```python
from build123d import *

# Parameters (mm, degrees)
SKETCH_1_R               = 13
EXTRUDE_1_DEPTH          = 8
SKETCH_2_R               = 17
EXTRUDE_2_DEPTH          = 8
EXTRUDE_3_DEPTH          = 8
SKETCH_4_R               = 13
EXTRUDE_4_DEPTH          = 6
SKETCH_5_R               = 10
CUT_EXTRUDE_1_DEPTH      = 25
SKETCH_7_R               = 2.5
CUT_EXTRUDE_3_DEPTH      = 32.5
PATTERN_CIRCULAR_1_COUNT = 2


with BuildPart() as part:
    # 草图1 → 凸台-拉伸1 (new body)
    with BuildSketch(Plane.XY):
        Circle(SKETCH_1_R)
    extrude(amount=EXTRUDE_1_DEPTH)

    # 草图2 → 凸台-拉伸2 (add)
    with BuildSketch(Plane(origin=(0, 0, 0), x_dir=(-1, 0, 0), z_dir=(0, 0, -1))):
        Circle(SKETCH_2_R)
    extrude(amount=EXTRUDE_2_DEPTH)

    # 草图3 → 凸台-拉伸3 (add)
    with BuildSketch(Plane.XY.offset(8)):
        with BuildLine():
            Line((2, 17.385338651), (17.385338651, 2))
            ThreePointArc((17.385338651, 2), (17.5, 0), (17.385338651, -2))
            Line((17.385338651, -2), (2, -17.385338651))
            ThreePointArc((2, -17.385338651), (0, -17.5), (-2, -17.385338651))
            Line((-2, -17.385338651), (-17.385338651, -2))
            ThreePointArc((-17.385338651, -2), (-17.5, 0), (-17.385338651, 2))
            Line((-17.385338651, 2), (-2, 17.385338651))
            ThreePointArc((-2, 17.385338651), (0, 17.5), (2, 17.385338651))
        make_face()
    extrude(amount=EXTRUDE_3_DEPTH)

    # 草图4 → 凸台-拉伸4 (add)
    with BuildSketch(Plane.XY.offset(16)):
        Circle(SKETCH_4_R)
    extrude(amount=EXTRUDE_4_DEPTH)

    # 草图5 → 切除-拉伸1 (cut)
    with BuildSketch(Plane(origin=(0, 0, -8), x_dir=(-1, 0, 0), z_dir=(0, 0, -1))):
        Circle(SKETCH_5_R)
    extrude(amount=-CUT_EXTRUDE_1_DEPTH, mode=Mode.SUBTRACT)

    # 草图7 → 切除-拉伸3 (cut)
    with BuildSketch(Plane.XY.offset(22)):
        with Locations((-6, 0)):
            Circle(SKETCH_7_R)
    cut_extrude_3 = extrude(amount=-CUT_EXTRUDE_3_DEPTH, mode=Mode.SUBTRACT)

    # 阵列(圆周)1: 切除-拉伸3 ×2 about axis
    pattern_circular_1_axis = Axis((0, 0, 0), (0, 0, 1))
    for i in range(1, PATTERN_CIRCULAR_1_COUNT):
        add(cut_extrude_3.rotate(pattern_circular_1_axis, i * 360 / PATTERN_CIRCULAR_1_COUNT), mode=Mode.SUBTRACT)


solid = part.part
```
Could you check a few things on this model? Use its own coordinates, in mm. A direction names the side the tool comes from. Coordinates: 2 decimals unless noted, no trailing zeros. Write each loop counter-clockwise with the first axis right and the second up, starting at its lowest first coordinate (ties: lowest second). Pieces come first, ordered by that corner, then holes. Notation, with made-up numbers: (24, 36) - (51, 36) arc R14 cw to (51, 40) - close; hole circle Ø6 at (-26, 7). An arc over 180 degrees is marked (long way). Use a Markdown table: item, result.
Q1. Imagine slicing it at B-B (y = -14). List the corners of the cut face in (x, z) for me, and give its area (3 significant figures).
Geometry check:
| item | result |
|---|---|
| outline | (-9.64, -8) - (9.64, -8) - (9.64, 0) - (-9.64, 0) - close; (-5.39, 8) - (5.39, 8) - (5.39, 16) - (-5.39, 16) - close |
| area | 240 mm2 |
Q2. Which directions (+Z, -Z, +X, -X, +Y, -Y) give clear straight access to the entire face, cutting with the end or side of a thin tool? Please do faces 1 (the cylindrical face through (-9.139, 14.334, -3.944)), 2 (the flat face through (-9.585, -9.8, 11.944)), 3 (the cylindrical face through (-10.316, -7.91, 18.958)), 4 (the flat face through (-9.8, 9.585, 11.944)), 5 (the flat face through (4, -13, 0)).
Geometry check:
| item | result |
|---|---|
| face 1 | -Z |
| face 2 | +Z, -X, -Y |
| face 3 | +Z |
| face 4 | +Z, -X, +Y |
| face 5 | none |
Q3. Please list where these lines run through material, in increasing order: L1, parallel to Z at x = 10, y = 8.5; L2, parallel to Z at x = 3.5, y = 8; L3, parallel to X at y = -7.5, z = -2.
Geometry check:
| item | result |
|---|---|
| L1 | z = -8 to 0, 8 to 16 |
| L2 | z = 17 to 22 |
| L3 | x = -15.26 to -6.61, 6.61 to 15.26 |
Q4. Thinking about a two-plate mould opening in X: for faces 6 (the cylindrical face through (2.17, -9.76, 4.32)), 7 (the flat face through (-3, -13, 16)), 8 (the flat face through (9.8, -9.585, 11.944)), which applies, +X half, -X half, draft (parallel to the pull), parting line (faces both ways), or undercut?
Geometry check:
| item | result |
|---|---|
| face 6 | undercut |
| face 7 | draft |
| face 8 | +X half |
Q5. Imagine slicing it at C-C (x = 0). List the corners of the cut face in (y, z) for me, and give its area (3 significant figures).
Geometry check:
| item | result |
|---|---|
| outline | (-17.5, 8) - (-13, 8) - (-13, 0) - (-17, 0) - (-17, -8) - (-10, -8) - (-10, 17) - (10, 17) - (10, -8) - (17, -8) - (17, 0) - (13, 0) - (13, 8) - (17.5, 8) - (17.5, 16) - (13, 16) - (13, 22) - (-13, 22) - (-13, 16) - (-17.5, 16) - close |
| area | 416 mm2 |
Q6. Imagine slicing it at D-D (x = 6). List the corners of the cut face in (y, z) for me.
Geometry check:
| item | result |
|---|---|
| outline | (-15.91, -8) - (-8, -8) - (-8, 17) - (-2.5, 17) - (-2.5, 22) - (-11.53, 22) - (-11.53, 16) - (-13.39, 16) - (-13.39, 8) - (-11.53, 8) - (-11.53, 0) - (-15.91, 0) - close; (2.5, 17) - (8, 17) - (8, -8) - (15.91, -8) - (15.91, 0) - (11.53, 0) - (11.53, 8) - (13.39, 8) - (13.39, 16) - (11.53, 16) - (11.53, 22) - (2.5, 22) - close |
Q7. Imagine slicing it at A-A (z = 14.5). List the corners of the cut face in (x, y) for me, and give its area (3 significant figures).
Geometry check:
| item | result |
|---|---|
| outline | (-17.39, -2) - (-2, -17.39) arc R17.5 ccw to (2, -17.39) - (17.39, -2) arc R17.5 ccw to (17.39, 2) - (2, 17.39) arc R17.5 ccw to (-2, 17.39) - (-17.39, 2) arc R17.5 ccw to start; hole circle Ø20 at (0, 0) |
| area | 423 mm2 |
Q8. I'm going to push flat-ended pins straight in: pin 1 Ø6 at (x, z) = (8, 16) entering from +Y; pin 2 Ø12 at (x, z) = (-5, 0.5) entering from -Y; pin 3 Ø3 at (x, z) = (-11, -4.5) entering from +Y; pin 4 Ø16 at (x, y) = (2, -2.5) entering from -Z. Where does each tip first touch, or does it pass through?
Geometry check:
| item | result |
|---|---|
| pin 1 | stops at y = 14.39 |
| pin 2 | stops at y = -17 |
| pin 3 | stops at y = 14.1 |
| pin 4 | stops at z = -8 |
